Verification items for the finished model (mm, model axes). Give positions to 0.01 mm unless a question says otherwise; leave off trailing zeros. Loops run counter-clockwise (first coordinate to the right, second up) from the corner with the lowest first, then second, coordinate; pieces in that order, holes last. Notation, with made-up numbers: (-6.5, 49.25) - (6.5, 49.25) arc R15 cw to (6.5, 72.25) - close; hole circle Ø3 at (-11.5, 35). An arc over 180 degrees is marked (long way). Answer in a Markdown table with one row per item.
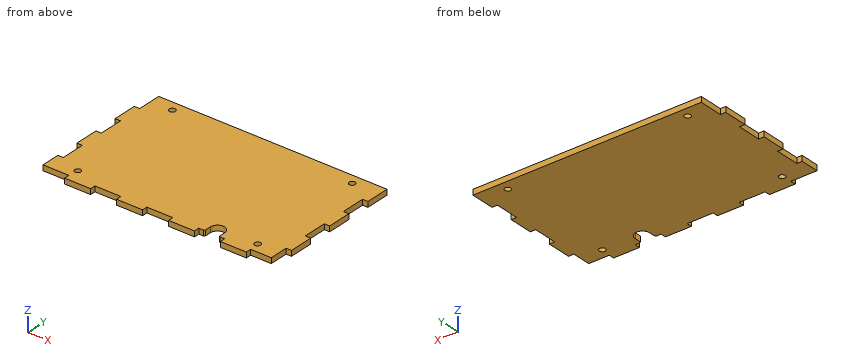
```python
from build123d import *

# Parameters (mm, degrees)
SKETCH1_W                      = 130
SKETCH1_H                      = 80
BOSS_EXTRUDE1_DEPTH            = 3
SKETCH2_W                      = 14.444444444
SKETCH2_H                      = 3
SKETCH2_W_2                    = 3
SKETCH2_H_2                    = 13.333333334
SKETCH2_H_3                    = 13.333333333
CUT_TABS_DEPTH                 = 153.672852859
CUT_CORNERPIECE_HOLES_REACH    = 154.673
SKETCH3_R                      = 1.7
CUT_POWER_CORD_CLEARANCE_REACH = 154.673
CHAMFER1_SIZE                  = 0.5


with BuildPart() as part:
    # Sketch1 → Boss-Extrude1 (new body)
    with BuildSketch(Plane.XY):
        with Locations((65, 40)):
            Rectangle(SKETCH1_W, SKETCH1_H)
    extrude(amount=BOSS_EXTRUDE1_DEPTH)

    # Sketch2 → Cut tabs (cut, through all)
    with BuildSketch(Plane.XY.offset(3)):
        with Locations((7.222222222, 1.5)):
            Rectangle(SKETCH2_W, SKETCH2_H)
        with Locations((36.111111111, 1.5)):
            Rectangle(SKETCH2_W, SKETCH2_H)
        with Locations((65, 1.5)):
            Rectangle(SKETCH2_W, SKETCH2_H)
        with Locations((93.888888889, 1.5)):
            Rectangle(SKETCH2_W, SKETCH2_H)
        Polygon((115.555555556, 0), (115.555555556, 3), (127, 3), (127, 13.333333333), (130, 13.333333333), (130, 0), align=None)
        with Locations((1.5, 20)):
            Rectangle(SKETCH2_W_2, SKETCH2_H_2)
        with Locations((1.5, 46.666666667)):
            Rectangle(SKETCH2_W_2, SKETCH2_H_3)
        with Locations((1.5, 73.333333334)):
            Rectangle(SKETCH2_W_2, SKETCH2_H_3)
        with Locations((128.5, 33.333333334)):
            Rectangle(SKETCH2_W_2, SKETCH2_H_3)
        with Locations((128.5, 60)):
            Rectangle(SKETCH2_W_2, SKETCH2_H_2)
    extrude(amount=-CUT_TABS_DEPTH, mode=Mode.SUBTRACT)

    # Sketch3 → Cut cornerpiece holes (cut, up to next)
    with BuildSketch(Plane.XY.offset(3), mode=Mode.PRIVATE) as cut_cornerpiece_holes_sk1:
        with Locations((15, 74.5)):
            Circle(SKETCH3_R)
    cut_cornerpiece_holes_tool1 = extrude(cut_cornerpiece_holes_sk1.sketch, amount=-CUT_CORNERPIECE_HOLES_REACH, mode=Mode.PRIVATE) & part.part
    # Sketch3 → Cut cornerpiece holes (cut, up to next)
    with BuildSketch(Plane.XY.offset(3), mode=Mode.PRIVATE) as cut_cornerpiece_holes_sk2:
        with Locations((115, 74.5)):
            Circle(SKETCH3_R)
    cut_cornerpiece_holes_tool2 = extrude(cut_cornerpiece_holes_sk2.sketch, amount=-CUT_CORNERPIECE_HOLES_REACH, mode=Mode.PRIVATE) & part.part
    # Sketch3 → Cut cornerpiece holes (cut, up to next)
    with BuildSketch(Plane.XY.offset(3), mode=Mode.PRIVATE) as cut_cornerpiece_holes_sk3:
        with Locations((15, 8.5)):
            Circle(SKETCH3_R)
    cut_cornerpiece_holes_tool3 = extrude(cut_cornerpiece_holes_sk3.sketch, amount=-CUT_CORNERPIECE_HOLES_REACH, mode=Mode.PRIVATE) & part.part
    # Sketch3 → Cut cornerpiece holes (cut, up to next)
    with BuildSketch(Plane.XY.offset(3), mode=Mode.PRIVATE) as cut_cornerpiece_holes_sk4:
        with Locations((115, 8.5)):
            Circle(SKETCH3_R)
    cut_cornerpiece_holes_tool4 = extrude(cut_cornerpiece_holes_sk4.sketch, amount=-CUT_CORNERPIECE_HOLES_REACH, mode=Mode.PRIVATE) & part.part
    add(cut_cornerpiece_holes_tool1.solids().sort_by_distance((15, 74.5, 3))[0], mode=Mode.SUBTRACT)
    add(cut_cornerpiece_holes_tool2.solids().sort_by_distance((115, 74.5, 3))[0], mode=Mode.SUBTRACT)
    add(cut_cornerpiece_holes_tool3.solids().sort_by_distance((15, 8.5, 3))[0], mode=Mode.SUBTRACT)
    add(cut_cornerpiece_holes_tool4.solids().sort_by_distance((115, 8.5, 3))[0], mode=Mode.SUBTRACT)

    # Sketch4 → Cut power cord clearance (cut, up to next)
    with BuildSketch(Plane(origin=(0, 0, 0), x_dir=(-1, 0, 0), z_dir=(0, 0, -1)), mode=Mode.PRIVATE) as cut_power_cord_clearance_sk1:
        with BuildLine():
            Line((-97.888888889, 3), (-97.888888889, 7))
            ThreePointArc((-97.888888889, 7), (-93.888888889, 11), (-89.888888889, 7))
            Line((-89.888888889, 7), (-89.888888889, 3))
            Line((-89.888888889, 3), (-97.888888889, 3))
        make_face()
    cut_power_cord_clearance_tool1 = extrude(cut_power_cord_clearance_sk1.sketch, amount=-CUT_POWER_CORD_CLEARANCE_REACH, mode=Mode.PRIVATE) & part.part
    add(cut_power_cord_clearance_tool1.solids().sort_by_distance((93.888889, 6.626601, 0))[0], mode=Mode.SUBTRACT)

    # Chamfer1
    chamfer1_edges = [part.edges().sort_by_distance(p)[0] for p in [
        (89.888888889, 3, 1.5),
        (97.888888889, 3, 1.5),
    ]]
    chamfer(chamfer1_edges, length=CHAMFER1_SIZE)


solid = part.part
```
Q1. Go/stop test with flat-tipped pins: P1, Ø1.5, axis at x = 122, z = 1.5, coming from the -Y side; P2, Ø1.5, axis at y = 8, z = 1.5, coming from the +X side. Record where each tip stops, or that it passes through.
Completed:
| item | result |
|---|---|
| P1 | y = 3 |
| P2 | x = 127 |
Q2. Sectioned sample at B-B (z = 0.6). Give the number of separate pieces and of enclosed holes in the cut face, and give its area (3 significant figures).
Completed:
| item | result |
|---|---|
| separate pieces | 1 |
| enclosed holes | 4 |
| area | 9,860 mm^2 |
Q3. Sectioned sample at A-A (y = 74.5). Record the cut outline in (x, z), and give its area (3 significant figures).
Completed:
| item | result |
|---|---|
| outline | (3, 0) - (13.3, 0) - (13.3, 3) - (3, 3) - close; (16.7, 0) - (113.3, 0) - (113.3, 3) - (16.7, 3) - close; (116.7, 0) - (130, 0) - (130, 3) - (116.7, 3) - close |
| area | 361 mm^2 |
Q4. Sectioned sample at D-D (x = 11). Record the cut outline in (y, z).
Completed:
| item | result |
|---|---|
| outline | (3, 0) - (80, 0) - (80, 3) - (3, 3) - close |
Q5. Sectioned sample at C-C (y = 30.5). Record the cut outline in (x, z).
Completed:
| item | result |
|---|---|
| outline | (0, 0) - (127, 0) - (127, 3) - (0, 3) - close |
Q6. Thickness scan on line 1 (X direction, y = 74.5, z = 0.95); line 2 (Y direction, x = 15, z = 0.65); line 3 (Y direction, x = 14, z = 1.6). Record the ranges inside material, lowest first.
Completed:
| item | result |
|---|---|
| line 1 | 3 to 13.3, 16.7 to 113.3, 116.7 to 130 |
| line 2 | 0 to 6.8, 10.2 to 72.8, 76.2 to 80 |
| line 3 | 3 to 7.13, 9.87 to 73.13, 75.87 to 80 |
